```python
from build123d import *

# Parameters (mm, degrees)
F1_DEPTH = 19.01698


with BuildPart() as f1:
    # F0 (on Right) → F1 (new body)
    with BuildSketch(Plane.YZ):
        with BuildLine():
            Line((-141.684375, -76.2), (136.462135, -76.2))
            Line((136.462135, -76.2), (136.462135, 44.45))
            ThreePointArc((136.462135, 44.45), (131.972007, 46.309872), (130.112135, 50.8))
            Line((130.112135, 50.8), (130.112135, 76.2))
            ThreePointArc((130.112135, 76.2), (-3.119611, 69.38236), (-135.334375, 51.59375))
            Line((-135.334375, 51.59375), (-135.334375, 25.4))
            ThreePointArc((-135.334375, 25.4), (-137.194247, 20.909872), (-141.684375, 19.05))
            Line((-141.684375, 19.05), (-141.684375, -76.2))
        make_face()
    extrude(amount=F1_DEPTH)


solid = f1.part
```
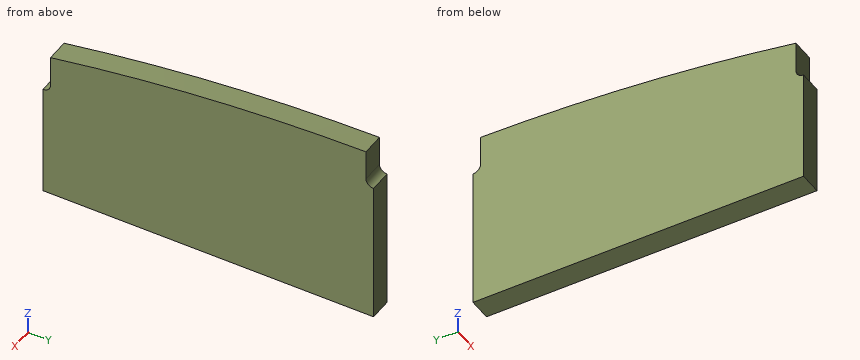
The model under review builds one solid part; all positions refer to its coordinate system, in mm. Round coordinates to 2 decimals unless told otherwise and drop trailing zeros. Loops run counter-clockwise (first coordinate to the right, second up) from the corner with the lowest first, then second, coordinate; pieces in that order, holes last. Notation, with made-up numbers: (-16.5, 76.5) - (9.5, 76.5) arc R24 cw to (9.5, 99.5) - close; hole circle Ø9 at (3.25, 81). An arc over 180 degrees is marked (long way). Use a Markdown table: item, result. Add a question column.
Q1. Add section A-A (x = 10.75). State the section outline as (y, z) points.
Q2. Insertion check: pin 1 Ø5.5 at (x, z) = (7, 67) entering from +Y; pin 2 Ø5.5 at (x, z) = (6, 44) entering from -Y. Each pin has a flat end and moves straight along its axis. Give the tip position at first contact, or say it passes through.
Q3. Add section C-C (y = -45.5). State the section outline as (x, z) points.
Q4. Add section B-B (z = 31.5). State the section outline as (x, y) points.
Q5. For probe 1 along Y at (x, z) = (9.5, 35.5); probe 2 along Z at (x, y) = (8.5, -118); probe 3 along Z at (x, y) = (17, 90), list the stretches that pass through material, from the lowest coordinate up.
Worked answers:
| question | item | result |
|---|---|---|
| 1 | outline | (-141.68, -76.2) - (136.46, -76.2) - (136.46, 44.45) arc R6.35 cw to (130.11, 50.8) - (130.11, 76.2) arc R1615.28 ccw to (-135.33, 51.59) - (-135.33, 25.4) arc R6.35 cw to (-141.68, 19.05) - close |
| 2 | pin 1 | y = 130.11 |
| 2 | pin 2 | y = -135.33 |
| 3 | outline | (0, -76.2) - (19.02, -76.2) - (19.02, 64.89) - (0, 64.89) - close |
| 4 | outline | (0, -135.33) - (19.02, -135.33) - (19.02, 136.46) - (0, 136.46) - close |
| 5 | probe 1 | -135.33 to 136.46 |
| 5 | probe 2 | -76.2 to 54.56 |
| 5 | probe 3 | -76.2 to 75.31 |
